Verification items for the finished model (mm, model axes). Face numbers are marked on the shaded views. A direction names the side the tool comes from. Coordinates: 2 decimals unless noted, no trailing zeros. Order: outer loops, then holes, each group sorted by start corner. A loop starts at its lowest first (then second) coordinate and runs counter-clockwise, first axis right, second up. Notation, with made-up numbers: (-10.75, 19.25) -> (27.25, 19.25) arc R18 cw to (27.25, 51.25) -> close; hole circle Ø8 at (-38.5, -28). An arc over 180 degrees is marked (long way). Write item = value, one per line. Start each with the question number.
from build123d import *

# Parameters (mm, degrees)
SKETCH1_W           = 350
SKETCH1_H           = 350
BOSS_EXTRUDE1_DEPTH = 50
SKETCH2_W           = 90
SKETCH2_H           = 90
BOSS_EXTRUDE2_DEPTH = 800
SKETCH3_W           = 60
SKETCH3_H           = 60
CUT_EXTRUDE1_DEPTH  = 800
SKETCH4_R           = 10
CUT_EXTRUDE3_DEPTH  = 221


with BuildPart() as part:
    # Sketch1 → Boss-Extrude1 (new body)
    with BuildSketch(Plane(origin=(0, 0, 0), x_dir=(1, 0, 0), z_dir=(0, 1, 0))):
        Rectangle(SKETCH1_W, SKETCH1_H)
    extrude(amount=BOSS_EXTRUDE1_DEPTH)

    # Sketch2 → Boss-Extrude2 (add)
    with BuildSketch(Plane(origin=(0, 50, 0), x_dir=(1, 0, 0), z_dir=(0, 1, 0))):
        Rectangle(SKETCH2_W, SKETCH2_H)
    extrude(amount=BOSS_EXTRUDE2_DEPTH)

    # Sketch3 → Cut-Extrude1 (cut)
    with BuildSketch(Plane(origin=(0, 850, 0), x_dir=(1, 0, 0), z_dir=(0, 1, 0))):
        Rectangle(SKETCH3_W, SKETCH3_H)
    extrude(amount=-CUT_EXTRUDE1_DEPTH, mode=Mode.SUBTRACT)

    # Sketch4 → Cut-Extrude3 (cut, through all)
    with BuildSketch(Plane.XY.offset(45)):
        with Locations((0, 830)):
            Circle(SKETCH4_R)
        with Locations((0, 770)):
            Circle(SKETCH4_R)
        with Locations((0, 710)):
            Circle(SKETCH4_R)
        with Locations((0, 650)):
            Circle(SKETCH4_R)
        with Locations((0, 590)):
            Circle(SKETCH4_R)
        with Locations((0, 530)):
            Circle(SKETCH4_R)
        with Locations((0, 470)):
            Circle(SKETCH4_R)
    extrude(amount=-CUT_EXTRUDE3_DEPTH, mode=Mode.SUBTRACT)


solid = part.part
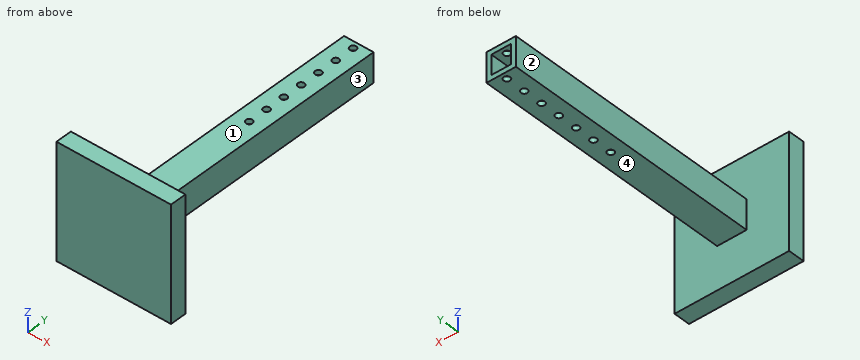
Item 1: Gauge pin test, flat ends, axial feed: P1, Ø6, axis at x = 1.5, y = 756.5, coming from the -Z side; P2, Ø18, axis at y = 328, z = 7, coming from the -X side; P3, Ø18, axis at x = 0, y = 710, coming from the +Z side; P4, Ø1, axis at x = 40.5, y = 399.5, coming from the +Z side. Record the tip position at first contact, or that the pin passes through.
Item 2: Section check A-A (y = 590). Record the boundary of the cut face in (x, z).
Item 3: Section check C-C (z = 132). Record the boundary of the cut face in (x, y), then the cut area to 3 significant figures.
Item 4: Section check B-B (x = 0). State how many separate pieces and enclosed holes the cut face has, then the cut area to 3 significant figures.
Item 5: Thickness scan on line 1 (Z direction, x = -28, y = 712); line 2 (X direction, y = 650, z = 39); line 3 (Y direction, x = 50, z = -101.5). Record the ranges inside material, lowest first.
Item 6: Tool access check on the marked faces 1, 2, 3 and 4. Record the directions out of +Z, -Z, +X, -X, +Y, -Y that give a thin tool (end or side, any length) a straight path to the whole face; none if there is none.
Filled sheet:
q1.P1 = -45
q1.P2 = -45
q1.P3 = through
q1.P4 = 45
q2.outline = (-45, -45) -> (-10, -45) -> (-10, -30) -> (-30, -30) -> (-30, 30) -> (-10, 30) -> (-10, 45) -> (-45, 45) -> close; (10, -45) -> (45, -45) -> (45, 45) -> (10, 45) -> (10, 30) -> (30, 30) -> (30, -30) -> (10, -30) -> close
q3.outline = (-175, 0) -> (175, 0) -> (175, 50) -> (-175, 50) -> close
q3.area = 17,500 mm^2
q4.separate_pieces = 15
q4.enclosed_holes = 0
q4.area = 37,300 mm^2
q5.line_1 = -45 to -30, 30 to 45
q5.line_2 = -45 to -10, 10 to 45
q5.line_3 = 0 to 50
q6.face_1 = +Z, +X, -X, +Y
q6.face_2 = +Z, -Z, -X, +Y
q6.face_3 = +Z, -Z, +X, +Y
q6.face_4 = -Z, +X, -X, +Y
